Autodesk Inventor part; units mm, degrees
ref_plane "YZ Plane" through (0, 0, 0) normal (1, 0, 0) x (0, 1, 0)
ref_plane "XZ Plane" through (0, 0, 0) normal (0, 1, 0) x (-1, 0, 0)
ref_plane "XY Plane" through (0, 0, 0) normal (0, 0, 1) x (1, 0, 0)
sketch "Sketch1" plane through (0, 0, 0) normal (0, 1, 0) x (-1, 0, 0)
  circle A0 centre (0, 0) radius 4.5
  circle A1 centre (0, 0) radius 10
  dimension "d0" = 9
  dimension "d1" = 20
extrude "Extrusion1" add sketch "Sketch1" along normal blind 3
sketch "Sketch2" plane through (0, 3, 0) normal (0, 1, 0) x (1, 0, 0)
  circle A0 centre (0, 0) radius 10
  circle A1 centre (0, 0) radius 10.5
  dimension "d4" = 21
extrude "Extrusion2" add sketch "Sketch2" against normal up to surface (3 mm away)
sketch "Sketch3" plane through (0, 3, 0) normal (0, 1, 0) x (1, 0, 0)
  circle A0 centre (0, 0) radius 12
  circle A1 centre (0, 0) radius 10.5
  dimension "d7" = 24
extrude "Extrusion3" add sketch "Sketch3" against normal up to surface (3 mm away)
properties part number "DedoAjuste"
Can you work these out from the model? Positions are in its coordinate system, mm. Coordinates: 2 decimals unless noted, no trailing zeros. Write each loop counter-clockwise with the first axis right and the second up, starting at its lowest first coordinate (ties: lowest second). Pieces come first, ordered by that corner, then holes. Notation, with made-up numbers: (30, 72.25) - (45, 72.25) arc R11 ccw to (45, 88.25) - close; hole circle Ø1 at (86, -0.75). An arc over 180 degrees is marked (long way). Return JSON: item names as keys, results as strings. Group by question number.
Item 1: If we section it at C-C (y = 1.6): Write out the boundary of the cut face in (x, z), then the cut area to 3 significant figures.
Item 2: We'd pull the mould along X, two halves only. Please class faces 1 (the face through (5, 0, 0)), 2 (the face through (-11.99, 1.52, -0.53)), 3 (the face through (0.59, 1.48, -4.46)): pulls with the +X half, pulls with the -X half, needs draft (parallel to the pull), parting line crosses it, or undercut.
Item 3: If we section it at D-D (z = 9.25): Write out the boundary of the cut face in (x, y).
Item 4: If we section it at B-B (z = 0): Write out the boundary of the cut face in (x, y).
Item 5: Please list where these lines run through material, in increasing order: probe 1 along Z at (x, y) = (0, 1.45); probe 2 along X at (y, z) = (2, 1.25); probe 3 along Z at (x, y) = (2.5, 1.05).
Item 6: I'm going to push flat-ended pins straight in: pin 1 Ø5.5 at (x, z) = (0, 0) entering from +Y; pin 2 Ø4 at (x, z) = (8, 7) entering from -Y; pin 3 Ø1.5 at (y, z) = (2.5, 9) entering from +X. Where does each tip first touch, or does it pass through?
Item 7: If we section it at A-A (x = 0): Write out the boundary of the cut face in (y, z).
Return value:
{
 "1": {"outline": "circle Ø24 at (0, 0); hole circle Ø9 at (0, 0)", "area": "389 mm^2"},
 "2": {"face 1": "needs draft", "face 2": "parting line crosses it", "face 3": "undercut"},
 "3": {"outline": "(-7.64, 0) - (7.64, 0) - (7.64, 3) - (-7.64, 3) - close"},
 "4": {"outline": "(-12, 0) - (-4.5, 0) - (-4.5, 3) - (-12, 3) - close; (4.5, 0) - (12, 0) - (12, 3) - (4.5, 3) - close"},
 "5": {"probe 1": "z = -12 to -4.5, 4.5 to 12", "probe 2": "x = -11.93 to -4.32, 4.32 to 11.93", "probe 3": "z = -11.74 to -3.74, 3.74 to 11.74"},
 "6": {"pin 1": "passes through", "pin 2": "stops at y = 0", "pin 3": "stops at x = 8.71"},
 "7": {"outline": "(0, -12) - (3, -12) - (3, -4.5) - (0, -4.5) - close; (0, 4.5) - (3, 4.5) - (3, 12) - (0, 12) - close"}
}
